Read the model definition and answer for the solid it produces. Units are mm, in the model's axes. A direction names the side the tool comes from. Coordinates: 2 decimals unless noted, no trailing zeros. Order: outer loops, then holes, each group sorted by start corner. A loop starts at its lowest first (then second) coordinate and runs counter-clockwise, first axis right, second up. Notation, with made-up numbers: M 37.25,12.25 L 91.25,12.25 A16 cw 91.25,32.25 Z; hole C -37.75,6 d9. An arc over 180 degrees is marked long. Use a Markdown table: item, result. Add a question column.
1) Find the intervals of material crossed by probe 1 along X at (y, z) = (-3.75, 0); probe 2 along X at (y, z) = (2, 0), in increasing order. Write a range as [from, to].
2) For faces 5 (the face through (6, -6.593, -6)), 6 (the face through (-2.579, -4.894, 1.978)), 7 (the face through (5.78, 7.31, -1.82)), determine the directions among +Z, -Z, +X, -X, +Y, -Y from which every point of the face is accessible in a straight line to the end or side of a thin tool.
3) Each of these flat-tipped pins is pushed along its axis until it touches: pin 1 Ø2 at (x, y) = (1, -3) entering from -Z; pin 2 Ø1 at (y, z) = (2, 2) entering from +X; pin 3 Ø10 at (y, z) = (1.5, 7) entering from +X. Where does it stop, or does it pass through?
4) Find section C-C on y = 8.5. Write down the section's boundary in (x, z).
5) Find section B-B on x = 0. Write down the section's boundary in (y, z).
6) Find section D-D on x = 11.5. Write down the section's boundary in (y, z), plus the area to 3 significant figures.
7) Find section A-A on z = 0. Write down the section's boundary in (x, y), plus the area to 3 significant figures.
8) The mould has two halves that part along Y. Classify faces 1 (the face through (-1.8, 10, 5.1)), 2 (the face through (0, -7, -13.782)), 3 (the face through (5.78, -4.45, -1.82)), 4 (the face through (-4.385, 1.509, -4.021)): released by +Y, released by -Y, zero draft, split by the parting line, or undercut.
from build123d import *

# Parameters (mm, degrees)
SKETCH2_OUTSIDE_W       = 53.884
SKETCH2_OUTSIDE_H       = 53.884
SKETCH2_OUTSIDE_W_2     = 28.986815524
SKETCH2_OUTSIDE_H_2     = 27.563826398
CUT_EXTRUDE1_DEPTH      = 11
CUT_EXTRUDE1_DEPTH_BACK = 9.193473012


with BuildPart() as part:
    # Sketch1 → Revolve1 (revolve)
    with BuildSketch(Plane.XY):
        Polygon((4.75, 9.5), (4.75, 0), (3.25, -1.5), (3.25, -8.193473012), (20, -8.193473012), (20, -6.593473012), (8.200842899, -6.593473012), (5.95, -4.342630114), (5.95, 7.2), (7.75, 9), (7.75, 10), (5.25, 10), align=None)
    revolve(axis=Axis((0, -12.923275862, 0), (0, 1, 0)))

    # Sketch2 outside → Cut-Extrude1 (cut, two sides)
    with BuildSketch(Plane(origin=(0, 0, 0), x_dir=(1, 0, 0), z_dir=(0, 1, 0))) as cut_extrude1_sk:
        Rectangle(SKETCH2_OUTSIDE_W, SKETCH2_OUTSIDE_H)
        Rectangle(SKETCH2_OUTSIDE_W_2, SKETCH2_OUTSIDE_H_2, mode=Mode.SUBTRACT)
    extrude(amount=CUT_EXTRUDE1_DEPTH, mode=Mode.SUBTRACT)
    extrude(cut_extrude1_sk.sketch, amount=-CUT_EXTRUDE1_DEPTH_BACK, mode=Mode.SUBTRACT)


solid = part.part
Check result:
| question | item | result |
|---|---|---|
| 1 | probe 1 | x = [-5.95, -3.25], [3.25, 5.95] |
| 1 | probe 2 | x = [-5.95, -4.75], [4.75, 5.95] |
| 2 | face 5 | +Y |
| 2 | face 6 | +Y, -Y |
| 2 | face 7 | none |
| 3 | pin 1 | stops at z = -5.95 |
| 3 | pin 2 | stops at x = 5.76 |
| 3 | pin 3 | stops at x = 5.6 |
| 4 | outline | C 0,0 d14.5; hole C 0,0 d9.5 |
| 5 | outline | M -8.19,-13.78 L -6.59,-13.78 L -6.59,-8.2 L -4.34,-5.95 L 7.2,-5.95 L 9,-7.75 L 10,-7.75 L 10,-5.25 L 9.5,-4.75 L 0,-4.75 L -1.5,-3.25 L -8.19,-3.25 Z; M -8.19,3.25 L -1.5,3.25 L 0,4.75 L 9.5,4.75 L 10,5.25 L 10,7.75 L 9,7.75 L 7.2,5.95 L -4.34,5.95 L -6.59,8.2 L -6.59,13.78 L -8.19,13.78 Z |
| 6 | outline | M -8.19,-13.78 L -6.59,-13.78 L -6.59,13.78 L -8.19,13.78 Z |
| 6 | area | 44.1 mm2 |
| 7 | outline | M -14.49,-8.19 L -3.25,-8.19 L -3.25,-1.5 L -4.75,0 L -4.75,9.5 L -5.25,10 L -7.75,10 L -7.75,9 L -5.95,7.2 L -5.95,-4.34 L -8.2,-6.59 L -14.49,-6.59 Z; M 3.25,-8.19 L 14.49,-8.19 L 14.49,-6.59 L 8.2,-6.59 L 5.95,-4.34 L 5.95,7.2 L 7.75,9 L 7.75,10 L 5.25,10 L 4.75,9.5 L 4.75,0 L 3.25,-1.5 Z |
| 7 | area | 105 mm2 |
| 8 | face 1 | released by +Y |
| 8 | face 2 | zero draft |
| 8 | face 3 | undercut |
| 8 | face 4 | undercut |
